Design review of the part shown in the three views and the two pictorial views. Dimensions are in mm from the part's minimum x, y and z. Round coordinates to 2 decimals unless told otherwise and drop trailing zeros. Order: outer loops, then holes, each group sorted by start corner. A loop starts at its lowest first (then second) coordinate and runs counter-clockwise, first axis right, second up. Notation, with made-up numbers: M 62.5,-15.5 L 68.5,-15.5 A20 cw 68.5,13.5 Z; hole C 70.25,11 d3. An arc over 180 degrees is marked long. Write item = value, one per line. Start each with the question number.
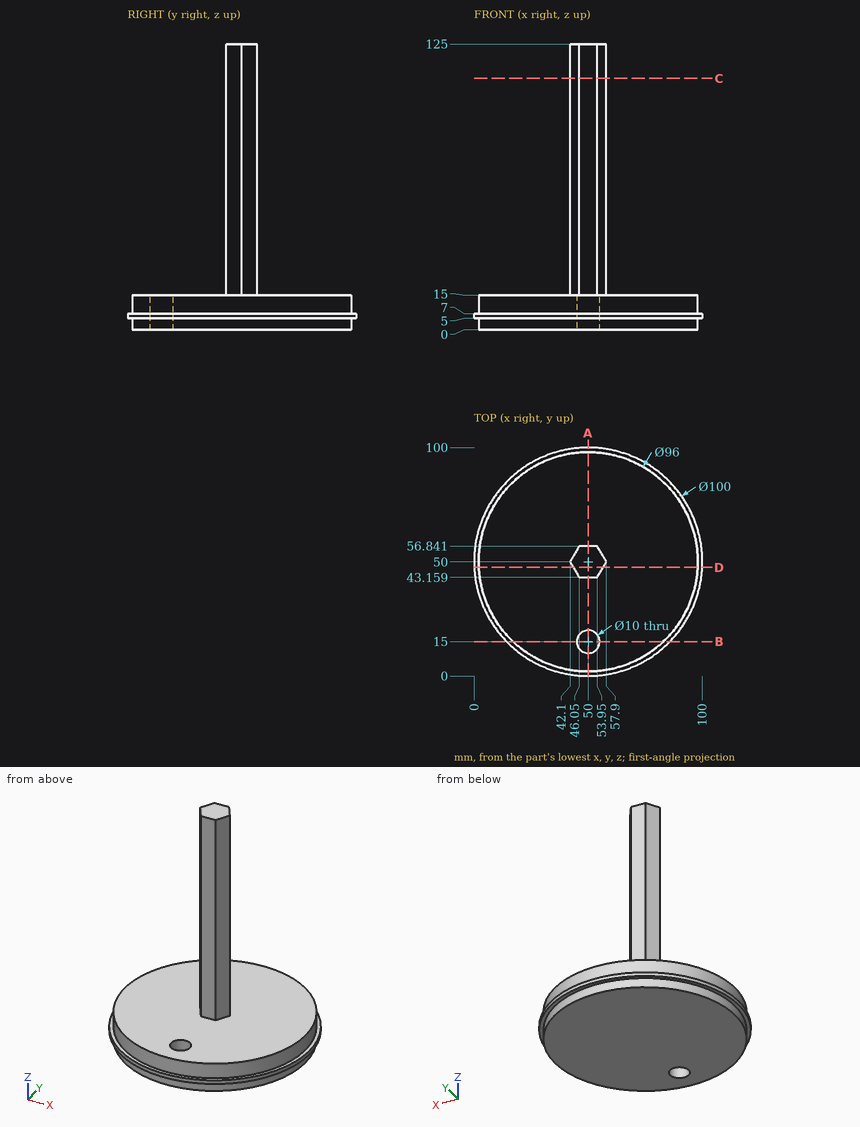
(1) We need section D-D, the plane y = 47.5. Write out the cut boundary in (x, z) (1 decimal).
(2) Insertion check: pin 1 (2.5 mm diameter, centred on x = 51.5, z = 73, fed in from -Y); pin 2 (10 mm diameter, centred on y = 25.5, z = 16, fed in from -X) (1 decimal); pin 3 (4 mm diameter, centred on x = 50, z = 59.5, fed in from +Y). Each pin has a flat end and moves straight along its axis. Give the tip position at first contact, or say it passes through.
(3) We need section A-A, the plane x = 50. Write out the cut boundary in (y, z), then the cut area to 3 significant figures.
(4) We need section C-C, the plane z = 110. Write out the cut boundary in (x, y), then the cut area to 3 significant figures.
(5) We need section B-B, the plane y = 15. Write out the cut boundary in (x, z), then the cut area to 3 significant figures.
(6) For line 1 along Y through (x, z) = (50, 9); line 2 along Z through (x, y) = (65.5, 50); line 3 along X through (y, z) = (15, 4.25), list the stretches that pass through material, from the lowest coordinate up.
Values:
q1.outline = M 0.1,5 L 2.1,5 L 2.1,0 L 97.9,0 L 97.9,5 L 99.9,5 L 99.9,7 L 97.9,7 L 97.9,15 L 56.5,15 L 56.5,125 L 43.5,125 L 43.5,15 L 2.1,15 L 2.1,7 L 0.1,7 Z
q2.pin_1 = 43.16
q2.pin_2 = 6.2
q2.pin_3 = 56.84
q3.outline = M 0,5 L 2,5 L 2,0 L 10,0 L 10,15 L 2,15 L 2,7 L 0,7 Z; M 20,0 L 98,0 L 98,5 L 100,5 L 100,7 L 98,7 L 98,15 L 56.84,15 L 56.84,125 L 43.16,125 L 43.16,15 L 20,15 Z
q3.area = 2,800 mm²
q4.outline = M 42.1,50 L 46.05,43.16 L 53.95,43.16 L 57.9,50 L 53.95,56.84 L 46.05,56.84 Z
q4.area = 162 mm²
q5.outline = M 14.29,5 L 17.15,5 L 17.15,0 L 45,0 L 45,15 L 17.15,15 L 17.15,7 L 14.29,7 Z; M 55,0 L 82.85,0 L 82.85,5 L 85.71,5 L 85.71,7 L 82.85,7 L 82.85,15 L 55,15 Z
q5.area = 847 mm²
q6.line_1 = 2 to 10, 20 to 98
q6.line_2 = 0 to 15
q6.line_3 = 17.15 to 45, 55 to 82.85
